The drawing under review shows one solid part. Ordinate dimensions are in mm from its lowest x, y, z. A direction names the side the tool comes from. Coordinates: 2 decimals unless noted, no trailing zeros. Order: outer loops, then holes, each group sorted by start corner. A loop starts at its lowest first (then second) coordinate and runs counter-clockwise, first axis right, second up. Notation, with made-up numbers: (42.25, 63) -> (88.25, 63) arc R24 ccw to (88.25, 76) -> close; hole circle Ø3 at (15, 80.25). An arc over 180 degrees is marked (long way). Put each result on its own line as item: value.
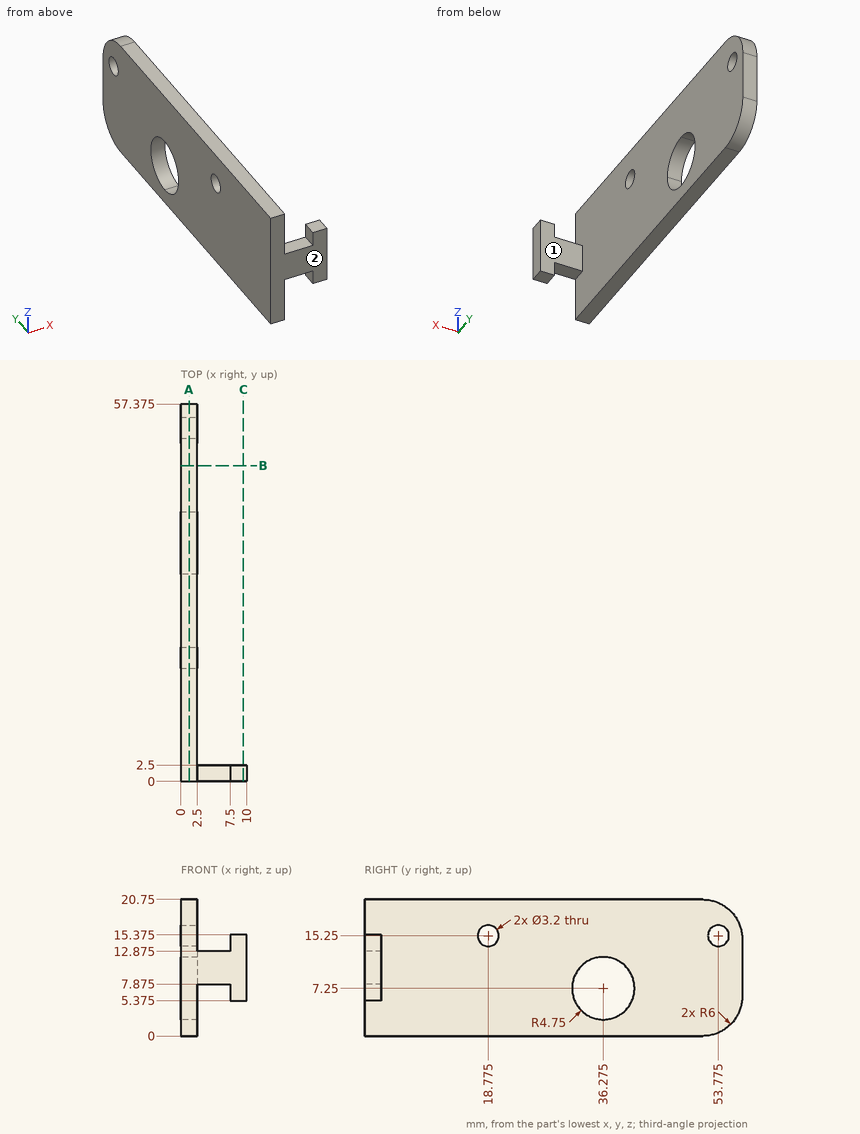
Item 1: For pin 1 Ø0.8 at (x, y) = (5.5, 1.5) entering from -Z (3 decimals); pin 2 Ø2 at (y, z) = (28.5, 13) entering from +X; pin 3 Ø3 at (x, y) = (9, 1) entering from +Z (3 decimals), all flat-tipped, find the tip position at first contact; note any pin that passes through.
Answers below:
pin 1: z = 7.875
pin 2: x = 2.5
pin 3: z = 15.375
Item 2: For the marked faces 1 and 2, list the 3-axis set-ups (+Z, -Z, +X, -X, +Y, -Y) from which the entire face can be reached by the end or side of a thin tool; tool diameter is ignored.
Answers below:
face 1: +Z, -Z, +X, +Y
face 2: +Z, -Z, +X, -X, -Y
Item 3: For line 1 (Y direction, x = 1.5, z = 15.25) (3 decimals); line 2 (X direction, y = 23.5, z = 1), list the stretches that pass through material, from the lowest coordinate up. Write a range as from..to.
Answers below:
line 1: 0..17.175, 20.375..52.175, 55.375..57.354
line 2: 0..2.5
Item 4: Consider section C-C on x = 9.5. Write out the cut boundary in (y, z) (3 decimals), and give its area (3 significant figures).
Answers below:
outline: (0, 5.375) -> (2.5, 5.375) -> (2.5, 15.375) -> (0, 15.375) -> close
area: 25.0 mm^2
Item 5: Consider section B-B on y = 48. Write out the cut boundary in (x, z).
Answers below:
outline: (0, 0) -> (2.5, 0) -> (2.5, 20.75) -> (0, 20.75) -> close
Item 6: Consider section A-A on x = 1.25. Write out the cut boundary in (y, z) (3 decimals), and give its area (3 significant figures).
Answers below:
outline: (0, 0) -> (51.375, 0) arc R6 ccw to (57.375, 6) -> (57.375, 14.75) arc R6 ccw to (51.375, 20.75) -> (0, 20.75) -> close; hole circle Ø3.2 at (18.775, 15.25); hole circle Ø9.5 at (36.275, 7.25); hole circle Ø3.2 at (53.775, 15.25)
area: 1,090 mm^2
